from build123d import *

# Parameters (mm, degrees)
SKETCH1_W           = 60
SKETCH1_H           = 10
BOSS_EXTRUDE1_DEPTH = 10
SKETCH2_W           = 40
SKETCH2_H           = 10
BOSS_EXTRUDE2_DEPTH = 40
SKETCH3_R           = 11
CUT_EXTRUDE1_DEPTH  = 8
SKETCH5_R           = 2
CUT_EXTRUDE2_DEPTH  = 45


with BuildPart() as part:
    # Sketch1 → Boss-Extrude1 (new body)
    with BuildSketch(Plane(origin=(0, 0, 0), x_dir=(1, 0, 0), z_dir=(0, 1, 0))):
        Rectangle(SKETCH1_W, SKETCH1_H)
    extrude(amount=BOSS_EXTRUDE1_DEPTH)

    # Sketch2 → Boss-Extrude2 (add)
    with BuildSketch(Plane(origin=(0, 10, 0), x_dir=(1, 0, 0), z_dir=(0, 1, 0))):
        Rectangle(SKETCH2_W, SKETCH2_H)
    extrude(amount=BOSS_EXTRUDE2_DEPTH)

    # Sketch3 → Cut-Extrude1 (cut)
    with BuildSketch(Plane(origin=(0, 0, -5), x_dir=(-1, 0, 0), z_dir=(0, 0, -1))):
        with Locations((0, 30)):
            Circle(SKETCH3_R)
    extrude(amount=-CUT_EXTRUDE1_DEPTH, mode=Mode.SUBTRACT)

    # Sketch5 → Cut-Extrude2 (cut)
    with BuildSketch(Plane(origin=(0, 10, 0), x_dir=(1, 0, 0), z_dir=(0, 1, 0))):
        with Locations(Location((-24.879663673, 0, 0), (0, 0, 270))):
            Circle(SKETCH5_R)
        with Locations(Location((25.342956813, 0, 0), (0, 0, 270))):
            Circle(SKETCH5_R)
    extrude(amount=-CUT_EXTRUDE2_DEPTH, mode=Mode.SUBTRACT)


solid = part.part
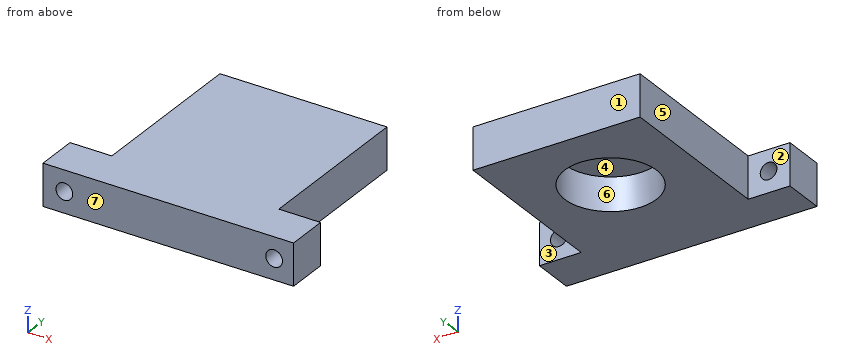
Build history of the part. All positions in model axes, mm. Face numbers are marked on the shaded views. A direction names the side the tool comes from. Round coordinates to 2 decimals unless told otherwise and drop trailing zeros. Write each loop counter-clockwise with the first axis right and the second up, starting at its lowest first coordinate (ties: lowest second). Pieces come first, ordered by that corner, then holes. Notation, with made-up numbers: (64.5, 43) -> (117.5, 43) arc R4 ccw to (117.5, 49) -> close; hole circle Ø10 at (-33.5, 30). An arc over 180 degrees is marked (long way). Use one line per item in the form item = value.
Q1. Drop flat-ended pins along their axis: P1, Ø3, axis at x = -23.5, z = -1, coming from the +Y side; P2, Ø5, axis at y = 20.5, z = 3, coming from the +X side; P3, Ø3.5, axis at x = 25.34, z = 0, coming from the +Y side; P4, Ø1, axis at y = 24.5, z = -2.5, coming from the -X side. Give the stop position or say it passes through.
Conclusion:
P1 = 10
P2 = 20
P3 = through
P4 = -20
Q2. Band-saw the part on A-A, the plane z = 0. Write the cut outline in (x, y), then the cut area to 3 significant figures.
Conclusion:
outline = (-30, 0) -> (-26.88, 0) -> (-26.88, 10) -> (-30, 10) -> close; (-22.88, 0) -> (23.34, 0) -> (23.34, 10) -> (20, 10) -> (20, 50) -> (-20, 50) -> (-20, 10) -> (-22.88, 10) -> close; (27.34, 0) -> (30, 0) -> (30, 10) -> (27.34, 10) -> close; hole circle Ø22 at (0, 30)
area = 1,740 mm²
Q3. Band-saw the part on D-D, the plane x = 7. Write the cut outline in (y, z).
Conclusion:
outline = (0, -5) -> (21.51, -5) -> (21.51, 3) -> (38.49, 3) -> (38.49, -5) -> (50, -5) -> (50, 5) -> (0, 5) -> close
Q4. Band-saw the part on B-B, the plane y = 30. Write the cut outline in (x, z), then the cut area to 3 significant figures.
Conclusion:
outline = (-20, -5) -> (-11, -5) -> (-11, 3) -> (11, 3) -> (11, -5) -> (20, -5) -> (20, 5) -> (-20, 5) -> close
area = 224 mm²
Q5. Band-saw the part on C-C, the plane z = -4. Write the cut outline in (x, y).
Conclusion:
outline = (-30, 0) -> (30, 0) -> (30, 10) -> (20, 10) -> (20, 50) -> (-20, 50) -> (-20, 10) -> (-30, 10) -> close; hole circle Ø22 at (0, 30)
Q6. Drill centre lines: L1, parallel to X at y = 6, z = 0; L2, parallel to Y at x = 0, z = 1.5; L3, parallel to X at y = 17, z = -1.75. Where is each one in solid material? Low to high.
Conclusion:
L1 = -30 to -26.88, -22.88 to 23.34, 27.34 to 30
L2 = 0 to 19, 41 to 50
L3 = -20 to 20
Q7. Tool access for the marked faces 1, 2 and 3: list every direction of +Z, -Z, +X, -X, +Y, -Y with a clear straight run to the whole face (end or side of a thin tool).
Conclusion:
face_1 = +Z, -Z, +X, -X, +Y
face_2 = +Z, -Z, -X, +Y
face_3 = +Z, -Z, +X, +Y
Q8. Two-plate mould, pull along Y, no slides. Class the marked faces 4, 5, 6 and 7: released by +Y, released by -Y, zero draft, split by the parting line, or undercut.
Conclusion:
face_4 = undercut
face_5 = zero draft
face_6 = undercut
face_7 = released by -Y
